```python
from build123d import *

# Parameters (mm, degrees)
F0_R     = 1.0365074283
F1_DEPTH = 5


with BuildPart() as f1:
    # F0 (on Top) → F1 (new body)
    with BuildSketch(Plane.XY):
        with BuildLine():
            ThreePointArc((-3.9841661922, 22.1444444444), (0, -22.5), (3.9841661922, 22.1444444444))
            ThreePointArc((3.9841661922, 22.1444444444), (0, 26.5), (-3.9841661922, 22.1444444444))
        make_face()
        with BuildLine():
            Line((-12.361779034, -3.8413735326), (-1.7917317985, -1.0537330189))
            add(Edge.make_bspline(
                [(-1.7917317985, -1.0537330189), (-1.5906673745, -1.8358674236), (-1.3134624845, -2.409225668)],
                knots=[5.3341932638, 5.3341932638, 5.3341932638, 5.6448500513, 5.6448500513, 5.6448500513], degree=2, weights=[1, 0.98796078, 1]))
            add(Edge.make_bspline(
                [(-1.3134624845, -2.409225668), (-19.5695791708, -9.1070002923), (-2.1141889978, -19.8879411926)],
                knots=[0.2281836428, 0.2281836428, 0.2281836428, 2.7689132091, 2.7689132091, 2.7689132091], degree=2, weights=[1, 0.2959324485, 1]))
            ThreePointArc((-2.1141889978, -19.8879411926), (-10.722049734, -16.8830580613), (-17.1017455245, -10.3696817702))
            Line((-17.1017455245, -10.3696817702), (-12.361779034, -3.8413735326))
        make_face(mode=Mode.SUBTRACT)
        with BuildLine():
            Line((-19.8736669699, 2.2444066409), (-2.1675859993, 1.4086192827))
            add(Edge.make_bspline(
                [(-2.1675859993, 1.4086192827), (-2.1191105118, 0.6776559948), (-2.0095094668, 0)],
                knots=[4.8951971827, 4.8951971827, 4.8951971827, 5.1359653729, 5.1359653729, 5.1359653729], degree=2, weights=[1, 0.9927625817, 1]))
            Line((-2.0095094668, 0), (-12.7543099225, -2.8337282129))
            Line((-12.7543099225, -2.8337282129), (-17.5429792365, -9.6043677308))
            ThreePointArc((-17.5429792365, -9.6043677308), (-19.6239577267, -3.8600884885), (-19.8736669699, 2.2444066409))
        make_face(mode=Mode.SUBTRACT)
        with BuildLine():
            add(Edge.make_bspline(
                [(2.1141889978, -19.8879411926), (19.5695791708, -9.1070002923), (1.3134624845, -2.409225668)],
                knots=[3.5142720981, 3.5142720981, 3.5142720981, 6.0550016644, 6.0550016644, 6.0550016644], degree=2, weights=[1, 0.2959324485, 1]))
            add(Edge.make_bspline(
                [(1.3134624845, -2.409225668), (1.5906673745, -1.8358674236), (1.7917317985, -1.0537330189)],
                knots=[0.6383352558, 0.6383352558, 0.6383352558, 0.9489920434, 0.9489920434, 0.9489920434], degree=2, weights=[1, 0.98796078, 1]))
            Line((1.7917317985, -1.0537330189), (12.361779034, -3.8413735326))
            Line((12.361779034, -3.8413735326), (17.1017455245, -10.3696817702))
            ThreePointArc((17.1017455245, -10.3696817702), (10.722049734, -16.8830580613), (2.1141889978, -19.8879411926))
        make_face(mode=Mode.SUBTRACT)
        with BuildLine():
            add(Edge.make_bspline(
                [(2.0095094668, 0), (2.1191105118, 0.6776559948), (2.1675859993, 1.4086192827)],
                knots=[1.1472199343, 1.1472199343, 1.1472199343, 1.3879881245, 1.3879881245, 1.3879881245], degree=2, weights=[1, 0.9927625817, 1]))
            Line((2.1675859993, 1.4086192827), (19.8736669699, 2.2444066409))
            ThreePointArc((19.8736669699, 2.2444066409), (19.6239577267, -3.8600884885), (17.5429792365, -9.6043677308))
            Line((17.5429792365, -9.6043677308), (12.7543099225, -2.8337282129))
            Line((12.7543099225, -2.8337282129), (2.0095094668, 0))
        make_face(mode=Mode.SUBTRACT)
        with BuildLine():
            Line((-13.1589546645, 15.0612719296), (-11.9581893981, 8.8521399225))
            Line((-11.9581893981, 8.8521399225), (-2.1184332771, 4.224274002))
            add(Edge.make_bspline(
                [(-2.1184332771, 4.224274002), (-2.2043163846, 3.3918710061), (-2.2043163846, 2.5257216766)],
                knots=[4.4323282948, 4.4323282948, 4.4323282948, 4.7123889804, 4.7123889804, 4.7123889804], degree=2, weights=[1, 0.9902117616, 1]))
            Line((-2.2043163846, 2.5257216766), (-19.7170367089, 3.3523817534))
            ThreePointArc((-19.7170367089, 3.3523817534), (-17.4494191733, 9.7733193192), (-13.1589546645, 15.0612719296))
        make_face(mode=Mode.SUBTRACT)
        with BuildLine():
            ThreePointArc((-12.0695648894, 15.9475892655), (-7.2930339661, 18.6228798946), (-1.9700282112, 19.9027382249))
            ThreePointArc((-1.9700282112, 19.9027382249), (-2.5376799412, 18.6867126776), (-2.0601059912, 17.4325716407))
            ThreePointArc((-2.0601059912, 17.4325716407), (-5.6475621585, 11.9263001397), (-1.6017195104, 6.7474947888))
            add(Edge.make_bspline(
                [(-1.6017195104, 6.7474947888), (-1.8617987609, 5.9806856047), (-2.0152058244, 5.0159234701)],
                knots=[3.9549946977, 3.9549946977, 3.9549946977, 4.2951442816, 4.2951442816, 4.2951442816], degree=2, weights=[1, 0.9855721107, 1]))
            Line((-2.0152058244, 5.0159234701), (-10.8698017311, 9.3490192993))
            Line((-10.8698017311, 9.3490192993), (-12.0695648894, 15.9475892655))
        make_face(mode=Mode.SUBTRACT)
        with Locations((-2.194955945, 14.6822528914)):
            Circle(F0_R, mode=Mode.SUBTRACT)
        with BuildLine():
            ThreePointArc((-1.0600310052, 19.9718886004), (0, 20), (1.0600310052, 19.9718886004))
            Line((1.0600310052, 19.9718886004), (1.0600310052, 17.7210549676))
            ThreePointArc((1.0600310052, 17.7210549676), (0, 17.8213354129), (-1.0600310052, 17.7210549676))
            Line((-1.0600310052, 17.7210549676), (-1.0600310052, 19.9718886004))
        make_face(mode=Mode.SUBTRACT)
        with BuildLine():
            ThreePointArc((-2.4961389938, 22.3611111111), (0, 25), (2.4961389938, 22.3611111111))
            ThreePointArc((2.4961389938, 22.3611111111), (0, 22.5), (-2.4961389938, 22.3611111111))
        make_face(mode=Mode.SUBTRACT)
        with BuildLine():
            add(Edge.make_bspline(
                [(2.2043163846, 2.5257216766), (2.2043163846, 3.3918710061), (2.1184332771, 4.224274002)],
                knots=[1.5707963268, 1.5707963268, 1.5707963268, 1.8508570124, 1.8508570124, 1.8508570124], degree=2, weights=[1, 0.9902117616, 1]))
            Line((2.1184332771, 4.224274002), (11.9581893981, 8.8521399225))
            Line((11.9581893981, 8.8521399225), (13.1589546645, 15.0612719296))
            ThreePointArc((13.1589546645, 15.0612719296), (17.4494191733, 9.7733193192), (19.7170367089, 3.3523817534))
            Line((19.7170367089, 3.3523817534), (2.2043163846, 2.5257216766))
        make_face(mode=Mode.SUBTRACT)
        with BuildLine():
            add(Edge.make_bspline(
                [(2.0152058244, 5.0159234701), (1.8617987609, 5.9806856047), (1.6017195104, 6.7474947888)],
                knots=[1.9880410256, 1.9880410256, 1.9880410256, 2.3281906095, 2.3281906095, 2.3281906095], degree=2, weights=[1, 0.9855721107, 1]))
            ThreePointArc((1.6017195104, 6.7474947888), (5.6475621585, 11.9263001397), (2.0601059912, 17.4325716407))
            ThreePointArc((2.0601059912, 17.4325716407), (2.5376799412, 18.6867126776), (1.9700282112, 19.9027382249))
            ThreePointArc((1.9700282112, 19.9027382249), (7.2930339661, 18.6228798946), (12.0695648894, 15.9475892655))
            Line((12.0695648894, 15.9475892655), (10.8698017311, 9.3490192993))
            Line((10.8698017311, 9.3490192993), (2.0152058244, 5.0159234701))
        make_face(mode=Mode.SUBTRACT)
        with Locations((2.194955945, 14.6822528914)):
            Circle(F0_R, mode=Mode.SUBTRACT)
    extrude(amount=F1_DEPTH)


solid = f1.part
```
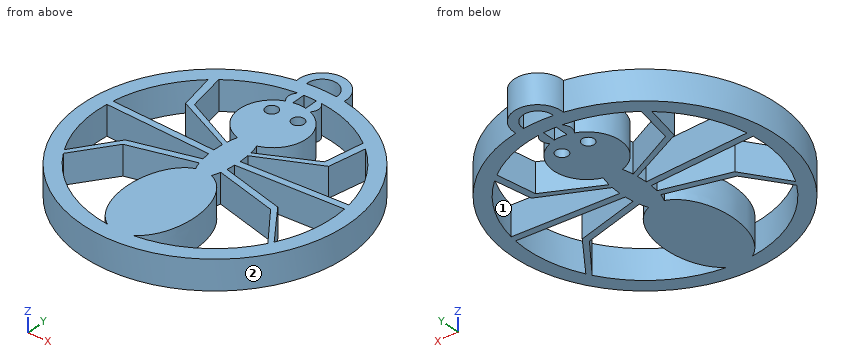
Part model, mm, in its own coordinate system. Face numbers are marked on the shaded views. Coordinates: 2 decimals unless noted, no trailing zeros. Order: outer loops, then holes, each group sorted by start corner. A loop starts at its lowest first (then second) coordinate and runs counter-clockwise, first axis right, second up. Notation, with made-up numbers: (39.25, 87.5) - (55.25, 87.5) arc R16 ccw to (55.25, 103.5) - close; hole circle Ø2 at (43, 44.25). An arc over 180 degrees is marked (long way). Return JSON: item names as keys, results as strings. Group by question number.
Item 1: Drill centre lines: probe 1 along X at (y, z) = (-4, 0.65); probe 2 along X at (y, z) = (12, 1.2); probe 3 along Y at (x, z) = (-14, 3.45) (3 decimals). Where is each one in solid material? Low to high. Write a range as from..to.
Item 2: Cut at C-C (z = 1.6). State how many separate pieces and enclosed holes the cut face has, plus the area to 3 significant figures.
Item 3: Cut at B-B (x = 9). List the corners of the cut face in (y, z), plus the area to 3 significant figures.
Item 4: Pull direction Y, two halves, no side cores. Call the marked faces 1 and 2: pulls with the +Y half, pulls with the -Y half, needs draft (parallel to the pull), parting line crosses it, or undercut.
Item 5: Cut at A-A (x = 0). List the corners of the cut face in (y, z).
Item 6: Pin check, flat tips, straight feed: pin 1 (1.9 mm diameter, centred on x = 2.19, y = 14.68, fed in from +Z); pin 2 (1.5 mm diameter, centred on y = 18.5, z = 3.5, fed in from -X); pin 3 (2 mm diameter, centred on x = -15.5, z = 3, fed in from +Y); pin 4 (1.1 mm diameter, centred on y = 19.5, z = 3, fed in from -X). Stop position of each tip, or through.
Check values:
{
 "1": {"probe 1": "x = -22.14..-19.6, -13.58..-12.48, -3.48..3.48, 12.48..13.58, 19.6..22.14", "probe 2": "x = -19.03..-16, -12.57..-11.35, -5.65..5.65, 11.35..12.57, 16..19.03", "probe 3": "y = -17.614..-14.283, -6.098..-4.595, 1.967..3.083, 14.283..17.614"},
 "2": {"separate pieces": "1", "enclosed holes": "12", "area": "761 mm2"},
 "3": {"outline": "(-20.62, 0) - (-17.86, 0) - (-17.86, 5) - (-20.62, 5) - close; (-2.95, 0) - (-1.84, 0) - (-1.84, 5) - (-2.95, 5) - close; (1.73, 0) - (2.85, 0) - (2.85, 5) - (1.73, 5) - close; (7.46, 0) - (8.43, 0) - (8.43, 5) - (7.46, 5) - close; (17.86, 0) - (20.62, 0) - (20.62, 5) - (17.86, 5) - close", "area": "43.6 mm2"},
 "4": {"face 1": "undercut", "face 2": "parting line crosses it"},
 "5": {"outline": "(-22.5, 0) - (17.82, 0) - (17.82, 5) - (-22.5, 5) - close; (20, 0) - (22.5, 0) - (22.5, 5) - (20, 5) - close; (25, 0) - (26.5, 0) - (26.5, 5) - (25, 5) - close"},
 "6": {"pin 1": "passes through", "pin 2": "stops at x = -13.83", "pin 3": "stops at y = 17.2", "pin 4": "stops at x = -12.13"}
}
